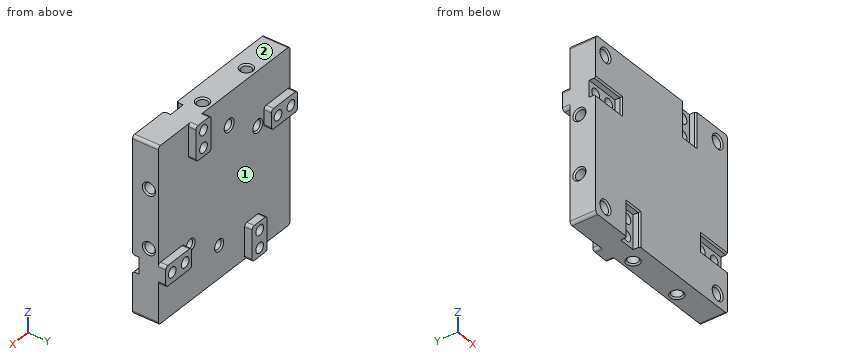
```python
from build123d import *

# Parameters (mm, degrees)
SKETCH1_W           = 61
SKETCH1_H           = 61
BOSS_EXTRUDE2_DEPTH = 9
SKETCH6_W           = 7
SKETCH6_H           = 12
SKETCH6_W_2         = 12
SKETCH6_H_2         = 7
BOSS_EXTRUDE4_DEPTH = 2.6
CIRPATTERN3_COUNT   = 4
SKETCH8_R           = 1.775
CUT_EXTRUDE3_DEPTH  = 45.666094524
CIRPATTERN4_COUNT   = 4
SKETCH10_W          = 11.9
SKETCH10_H          = 5.8
SKETCH10_W_2        = 5.8
SKETCH10_H_2        = 11.9
CUT_EXTRUDE6_DEPTH  = 2.3
SKETCH12_R          = 2.05
CUT_EXTRUDE8_DEPTH  = 6.5
FILLET1_R           = 1
SKETCH14_R          = 1.8
CUT_EXTRUDE10_DEPTH = 6.5
CIRPATTERN5_COUNT   = 4
CHAMFER1_SIZE       = 0.5
SKETCH16_R          = 1.8
CUT_EXTRUDE11_DEPTH = 6.5
SKETCH18_R          = 1.6
CUT_EXTRUDE12_DEPTH = 4.5
CHAMFER2_SIZE       = 0.5


with BuildPart() as part:
    # Sketch1 → Boss-Extrude2 (new body)
    with BuildSketch(Plane(origin=(0, 0, 0), x_dir=(1, 0, 0), z_dir=(0, 1, 0))):
        Rectangle(SKETCH1_W, SKETCH1_H)
    extrude(amount=BOSS_EXTRUDE2_DEPTH)

    # Sketch6 → Boss-Extrude4 (add)
    with BuildSketch(Plane(origin=(0, 9, 0), x_dir=(1, 0, 0), z_dir=(0, 1, 0))):
        with Locations((13, -24.5)):
            Rectangle(SKETCH6_W, SKETCH6_H)
        with Locations((24.5, 13)):
            Rectangle(SKETCH6_W_2, SKETCH6_H_2)
    boss_extrude4 = extrude(amount=BOSS_EXTRUDE4_DEPTH)

    # CirPattern3: Boss-Extrude4 ×4 about axis
    cirpattern3_axis = Axis((0, 0, 0), (0, 1, 0))
    for i in range(1, CIRPATTERN3_COUNT):
        add(boss_extrude4.rotate(cirpattern3_axis, i * 360 / CIRPATTERN3_COUNT))

    # Sketch8 → Cut-Extrude3 (cut, through all)
    with BuildSketch(Plane(origin=(0, 11.6, 0), x_dir=(1, 0, 0), z_dir=(0, 1, 0))):
        with Locations(Location((13, -21.5, 0), (0, 0, 270))):
            Circle(SKETCH8_R)
        with Locations(Location((13, -27.5, 0), (0, 0, 270))):
            Circle(SKETCH8_R)
    cut_extrude3 = extrude(amount=-CUT_EXTRUDE3_DEPTH, mode=Mode.SUBTRACT)

    # CirPattern4: Cut-Extrude3 ×4 about axis
    cirpattern4_axis = Axis((0, 0, 0), (0, 1, 0))
    for i in range(1, CIRPATTERN4_COUNT):
        add(cut_extrude3.rotate(cirpattern4_axis, i * 360 / CIRPATTERN4_COUNT), mode=Mode.SUBTRACT)

    # Sketch10 → Cut-Extrude6 (cut)
    with BuildSketch(Plane.XZ):
        with Locations((-24.55, 13)):
            Rectangle(SKETCH10_W, SKETCH10_H)
        with Locations((13, 24.55)):
            Rectangle(SKETCH10_W_2, SKETCH10_H_2)
        with Locations((24.55, -13)):
            Rectangle(SKETCH10_W, SKETCH10_H)
        with Locations((-13, -24.55)):
            Rectangle(SKETCH10_W_2, SKETCH10_H_2)
    extrude(amount=-CUT_EXTRUDE6_DEPTH, mode=Mode.SUBTRACT)

    # Sketch12 → Cut-Extrude8 (cut)
    with BuildSketch(Plane.XZ):
        with Locations(Location((-26, 26, 0), (0, 0, 270))):
            Circle(SKETCH12_R)
        with Locations(Location((26, 26, 0), (0, 0, 270))):
            Circle(SKETCH12_R)
        with Locations(Location((-26, -26, 0), (0, 0, 270))):
            Circle(SKETCH12_R)
        with Locations(Location((26, -26, 0), (0, 0, 270))):
            Circle(SKETCH12_R)
    extrude(amount=-CUT_EXTRUDE8_DEPTH, mode=Mode.SUBTRACT)

    # Fillet1
    fillet1_edges = [part.edges().sort_by_distance(p)[0] for p in [
        (30.5, 10.3, -9.5),
        (30.5, 10.3, -16.5),
        (18.5, 10.3, -16.5),
        (18.5, 10.3, -9.5),
        (9.5, 10.3, 18.5),
        (9.5, 10.3, 30.5),
        (16.5, 10.3, 30.5),
        (16.5, 10.3, 18.5),
        (-18.5, 10.3, 9.5),
        (-30.5, 10.3, 9.5),
        (-30.5, 10.3, 16.5),
        (-18.5, 10.3, 16.5),
        (-9.5, 10.3, -18.5),
        (-9.5, 10.3, -30.5),
        (-16.5, 10.3, -30.5),
        (-16.5, 10.3, -18.5),
        (-30.5, 4.5, -30.5),
        (30.5, 4.5, -30.5),
        (30.5, 4.5, 30.5),
        (-30.5, 4.5, 30.5),
    ]]
    fillet(fillet1_edges, radius=FILLET1_R)

    # Sketch14 → Cut-Extrude10 (cut)
    with BuildSketch(Plane.XY.offset(30.5)):
        with Locations((-14.66, 5.71)):
            Circle(SKETCH14_R)
        with Locations((5.66, 5.71)):
            Circle(SKETCH14_R)
    cut_extrude10 = extrude(amount=-CUT_EXTRUDE10_DEPTH, mode=Mode.SUBTRACT)

    # CirPattern5: Cut-Extrude10 ×4 about axis
    cirpattern5_axis = Axis((0, 0, 0), (0, 1, 0))
    for i in range(1, CIRPATTERN5_COUNT):
        add(cut_extrude10.rotate(cirpattern5_axis, i * 360 / CIRPATTERN5_COUNT), mode=Mode.SUBTRACT)

    # Chamfer1
    chamfer1_edges = [part.edges().sort_by_distance(p)[0] for p in [
        (-24.55, 0, 10.1),
        (-18.6, 0, 13),
        (-24.55, 0, 15.9),
        (10.1, 0, 24.55),
        (13, 0, 18.6),
        (15.9, 0, 24.55),
        (24.55, 0, -10.1),
        (18.6, 0, -13),
        (24.55, 0, -15.9),
        (-10.1, 0, -24.55),
        (-13, 0, -18.6),
        (-15.9, 0, -24.55),
        (-26, 0, 28.05),
        (-26, 0, -23.95),
        (26, 0, -23.95),
        (26, 0, 28.05),
        (-16.46, 5.71, 30.5),
        (3.86, 5.71, 30.5),
        (30.5, 5.71, 16.46),
        (30.5, 5.71, -3.86),
        (16.46, 5.71, -30.5),
        (-3.86, 5.71, -30.5),
        (-30.5, 5.71, -16.46),
        (-30.5, 5.71, 3.86),
    ]]
    chamfer(chamfer1_edges, length=CHAMFER1_SIZE)

    # Sketch16 → Cut-Extrude11 (cut)
    with BuildSketch(Plane(origin=(0, 9, 0), x_dir=(1, 0, 0), z_dir=(0, 1, 0))):
        with Locations(Location((-15.632217848, -11.576300085, 0), (0, 0, 270))):
            Circle(SKETCH16_R)
        with Locations(Location((-2.335254394, -19.285234053, 0), (0, 0, 270))):
            Circle(SKETCH16_R)
    extrude(amount=-CUT_EXTRUDE11_DEPTH, mode=Mode.SUBTRACT)

    # Sketch18 → Cut-Extrude12 (cut)
    with BuildSketch(Plane(origin=(0, 9, 0), x_dir=(1, 0, 0), z_dir=(0, 1, 0))):
        with Locations(Location((15.5, 11.478387332, 0), (0, 0, 270))):
            Circle(SKETCH18_R)
        with Locations(Location((2.315502731, 19.122118865, 0), (0, 0, 270))):
            Circle(SKETCH18_R)
    extrude(amount=-CUT_EXTRUDE12_DEPTH, mode=Mode.SUBTRACT)

    # Chamfer2
    chamfer2_edges = [part.edges().sort_by_distance(p)[0] for p in [
        (-15.632217848, 9, 9.776300085),
        (-2.335254394, 9, 17.485234053),
        (15.5, 9, -13.078387332),
        (2.315502731, 9, -20.722118865),
    ]]
    chamfer(chamfer2_edges, length=CHAMFER2_SIZE)


solid = part.part
```
Can you work these out from the model? Positions are in its coordinate system, mm. Face numbers are marked on the shaded views. A direction names the side the tool comes from. Coordinates: 2 decimals unless noted, no trailing zeros. Write each loop counter-clockwise with the first axis right and the second up, starting at its lowest first coordinate (ties: lowest second). Pieces come first, ordered by that corner, then holes. Notation, with made-up numbers: M 43,-20.75 L 74,-20.75 A23 ccw 74,14.25 Z; hole C -11.75,40 d7. An arc over 180 degrees is marked long. Write item = value, one per line. Start each with the question number.
Q1. If I drill on L1, parallel to Y at x = -26, z = -14.5; L2, parallel to X at y = 8.5, z = 10; L3, parallel to Z at x = 26.5, y = 2.75, over which ranges is the centre line in solid material (lowest first)? Write a range as [from, to].
Q2. If we section it at C-C, the plane y = 10.75: State how many separate pieces and enclosed holes the cut face has, then the cut area to 3 significant figures.
Q3. If we section it at B-B, the plane z = -5.66: Write out the boundary of the cut face in (x, y), then the cut area to 3 significant figures.
Q4. If we section it at A-A, the plane x = 21.5: Write out the boundary of the cut face in (y, z) (3 decimals), then the cut area to 3 significant figures.
Q5. On a 3-axis mill with a long thin cutter (end or side, diameter ignored), from which of +Z, -Z, +X, -X, +Y, -Y can I reach the whole of each face in a straight line? I mean the marked faces 1 and 2. Say none if no direction works.
Q6. I'm going to push flat-ended pins straight in: pin 1 (1 mm diameter, centred on x = 2, z = -19, fed in from +Y); pin 2 (4 mm diameter, centred on x = 2.32, z = -19.12, fed in from +Y) (3 decimals); pin 3 (2 mm diameter, centred on x = 13, z = 21.5, fed in from +Y); pin 4 (1 mm diameter, centred on x = 1.5, z = 11, fed in from +Y). Where does each tip first touch, or does it pass through?
Check sheet entries:
q1.L1 = [0, 3.92], [7.5, 9]
q1.L2 = [-30.5, -16.5], [-14.76, 30.5]
q1.L3 = [-30.5, -27.99], [-24.01, -14.47], [-11.53, 24.01], [27.99, 30.5]
q2.separate_pieces = 4
q2.enclosed_holes = 8
q2.area = 253 mm²
q3.outline = M -30.5,0 L 30.5,0 L 30.5,3.41 L 30,3.91 L 24,3.91 L 24,7.51 L 30,7.51 L 30.5,8.01 L 30.5,9 L -30.5,9 Z
q3.area = 525 mm²
q4.outline = M 0,-30.5 L 9,-30.5 L 9,-16.5 L 11.6,-16.5 L 11.6,-14.775 L 2.3,-14.775 L 2.3,-15.9 L 0.5,-15.9 L 0,-16.4 Z; M 0,-9.6 L 0.5,-10.1 L 2.3,-10.1 L 2.3,-11.225 L 11.6,-11.225 L 11.6,-9.5 L 9,-9.5 L 9,30.5 L 0,30.5 Z
q4.area = 521 mm²
q5.face_1 = +Y
q5.face_2 = +Z, +X, -X, +Y, -Y
q6.pin_1 = 4.5
q6.pin_2 = 8.905
q6.pin_3 = through
q6.pin_4 = 9
